Geometry: see drawing. Coordinates: mm, zero at the bounding-box minimum. Give positions to 0.01 mm unless a question says otherwise; leave off trailing zeros. Write each loop counter-clockwise with the first axis right and the second up, starting at its lowest first coordinate (ties: lowest second). Pieces come first, ordered by that corner, then holes. Notation, with made-up numbers: (-2.75, 86.5) -> (48.25, 86.5) arc R25 cw to (48.25, 109.5) -> close; hole circle Ø11 at (59.5, 14.5). An arc over 180 degrees is marked (long way). Use CSV: the item, a comma, the result in double quotes. Start each with the question number.
1) Section A-A (x = 9.5). Output: boundary loops of the cut face in (y, z).
2) Material intervals for line 1 (Y direction, x = 8, z = 4.25); line 2 (Y direction, x = 65.5, z = 6.5); line 3 (X direction, y = 6.75, z = 1.25), sorted ascending. Write a range as [from, to].
3) Contact query for flat-ended pins moving along their axis: P1, Ø3, axis at x = 58.5, y = 1, coming from the -Z side; P2, Ø4, axis at x = 8, y = 1, coming from the +Z side; P3, Ø4, axis at x = 54, y = 1.5, coming from the -Z side. Output: stop coordinate, or through.
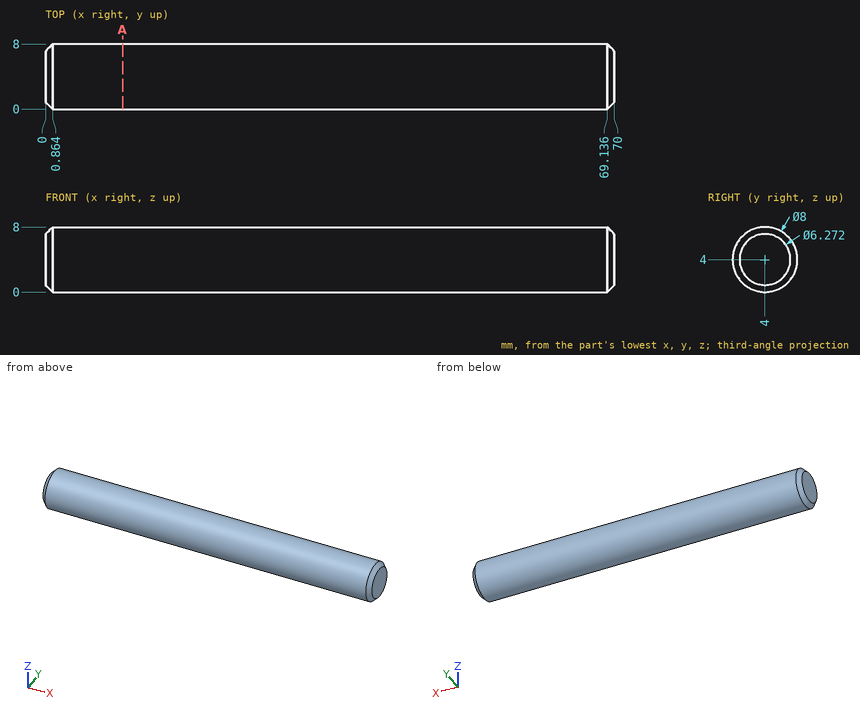
Answers follow:
1,outline,"circle Ø8 at (4, 4)"
2,line 1,"y = [0.01, 7.99]"
2,line 2,"y = [0.88, 7.12]"
2,line 3,"x = [0.75, 69.25]"
3,P1,"stops at z = 0.29"
3,P2,"stops at z = 7.87"
3,P3,"stops at z = 0.03"
